Input: part model. Units: mm. Frame: model coordinates. A direction names the side the tool comes from. Coordinates: 2 decimals unless noted, no trailing zeros. Loops run counter-clockwise (first coordinate to the right, second up) from the corner with the lowest first, then second, coordinate; pieces in that order, holes last.
Item 1: Pull-direction query (Y, two-part tool) for faces 3 (the flat face through (-147, 305, 15.875)), 4 (the flat face through (165.424, 142.991, 7.826)), 5 (the flat face through (155.993, 141.57, 9.392)); classes: released by +Y, released by -Y, zero draft, split by the parting line, or undercut.
Item 2: Ray query, line 1 along X through (y, z) = (147.5, 16); line 2 along Y through (x, z) = (25, 8.75); line 3 along X through (y, z) = (29.5, 9.5). Return the intervals inside material, ascending.
Item 3: Reachability of faces 1 (the flat face through (-133.66, 416.26, 17.44)), 2 (the flat face through (-138.43, 416.8, 7.83)) from +Z, -Z, +X, -X, +Y, -Y: full face, straight path, thin tool, end or side. Return the list, or none.
Item 4: Section A-A on y = 627. Return loops of the section in (x, z) (3 decimals), and give its area (3 significant figures).
Item 5: Contact query for flat-ended pins moving along their axis: P1, Ø4, axis at x = 102.5, z = 14.5, coming from the -Y side; P2, Ø8, axis at y = 276.5, z = 16, coming from the +X side; P3, Ø10, axis at x = 84.5, z = 12, coming from the -Y side. Output: stop coordinate, or through.
```python
from build123d import *

# Parameters (mm, degrees)
BOSS_EXTRUDE1_DEPTH = 19.05
CUT_EXTRUDE1_START  = -3.175
CUT_EXTRUDE1_DEPTH  = 3.175


# Read off the part's stored shape, not the designer's step: Cut-Extrude1
with BuildPart() as part:
    # Sketch1 → Boss-Extrude1 (new body)
    with BuildSketch(Plane.XY):
        with BuildLine():
            Line((157.234081882, 128.980548454), (154.716315658, 154.51789158))
            Line((154.716315658, 154.51789158), (164.195357535, 155.452445004))
            Line((164.195357535, 155.452445004), (166.6875, 130.175))
            add(Edge.make_bspline(
                [(0, 0), (73.666580622, 1.740675992), (181.188092361, 36.200835609), (166.6875, 130.175)],
                knots=[0, 0, 0, 0, 1, 1, 1, 1], degree=3))
            add(Edge.make_bspline(
                [(0, 0), (-73.666580622, 1.740675992), (-181.188092361, 36.200835609), (-166.6875, 130.175)],
                knots=[0, 0, 0, 0, 1, 1, 1, 1], degree=3))
            Line((-166.6875, 130.175), (-109.368223301, 711.556235093))
            Line((-109.368223301, 711.556235093), (-99.889181424, 710.621681669))
            Line((-99.889181424, 710.621681669), (-157.234081882, 128.980548454))
            add(Edge.make_bspline(
                [(0, 9.52776174), (-1.117611602, 9.555193192), (-3.340472897, 9.624755056), (-7.880039481, 9.827207732), (-13.652210416, 10.198958437), (-20.725459036, 10.840441372), (-30.303235723, 11.962316267), (-42.47749757, 13.875858033), (-57.165232888, 17.02314898), (-71.689613059, 21.050850851), (-90.515854195, 27.626537064), (-112.436111514, 38.157452487), (-130.643933928, 51.803557723), (-142.189146149, 64.564536934), (-149.192253507, 75.075537554), (-153.541361304, 84.674022673), (-156.058613173, 92.923629982), (-157.442658539, 99.418206789), (-158.29640922, 106.242287005), (-158.540175044, 112.221426054), (-158.437150466, 117.190167219), (-158.20642164, 121.010360535), (-157.881730698, 124.277278241), (-157.584058118, 126.601085874), (-157.415798733, 127.781927866), (-157.316566229, 128.446705395), (-157.261207353, 128.804756083), (-157.234081882, 128.980548454)],
                knots=[0.001057036, 0.001057036, 0.001057036, 0.001057036, 0.016679825, 0.032302613, 0.063548191, 0.094793768, 0.126039346, 0.1885305, 0.251021655, 0.31351281, 0.376003965, 0.500986274, 0.625968584, 0.688459739, 0.750950893, 0.813442048, 0.844687626, 0.875933203, 0.90717878, 0.938424358, 0.954047147, 0.969669935, 0.985292724, 0.993104118, 0.997009815, 0.998962664, 1.000915513, 1.000915513, 1.000915513, 1.000915513], degree=3))
            add(Edge.make_bspline(
                [(157.234081882, 128.980548454), (157.261207353, 128.804756083), (157.316566229, 128.446705395), (157.415798733, 127.781927866), (157.584058118, 126.601085874), (157.881730698, 124.277278241), (158.20642164, 121.010360535), (158.437150466, 117.190167219), (158.540175044, 112.221426054), (158.29640922, 106.242287005), (157.442658539, 99.418206789), (156.058613173, 92.923629982), (153.541361304, 84.674022673), (149.192253507, 75.075537554), (142.189146149, 64.564536934), (130.643933928, 51.803557723), (112.436111514, 38.157452487), (90.515854195, 27.626537064), (71.689613059, 21.050850851), (57.165232888, 17.02314898), (42.47749757, 13.875858033), (30.303235723, 11.962316267), (20.725459036, 10.840441372), (13.652210416, 10.198958437), (7.880039481, 9.827207732), (3.340472897, 9.624755056), (1.117611602, 9.555193192), (0, 9.52776174)],
                knots=[0.001057036, 0.001057036, 0.001057036, 0.001057036, 0.003009885, 0.004962733, 0.00886843, 0.016679825, 0.032302613, 0.047925402, 0.063548191, 0.094793768, 0.126039346, 0.157284923, 0.1885305, 0.251021655, 0.31351281, 0.376003965, 0.500986274, 0.625968584, 0.688459739, 0.750950893, 0.813442048, 0.875933203, 0.90717878, 0.938424358, 0.969669935, 0.985292724, 1.000915513, 1.000915513, 1.000915513, 1.000915513], degree=3))
        make_face()
    extrude(amount=BOSS_EXTRUDE1_DEPTH)

    # Cut-Extrude1 outline → Cut-Extrude1 (cut)
    with BuildSketch(Plane.XY.offset(19.05).offset(CUT_EXTRUDE1_START)):
        with BuildLine():
            add(Edge.make_bspline(
                [(0, 4.801965673), (9.039076986, 5.019645615), (18.615343357, 5.740087083), (38.206551494, 8.290420977), (48.221803102, 10.120302171), (68.063126794, 14.983315661), (77.889169822, 18.016665839), (96.726604846, 25.367412999), (105.737388343, 29.685039413), (122.329339782, 39.664160586), (129.908900725, 45.324695844), (139.777007016, 54.855777785), (142.816728459, 58.206110887), (148.333510848, 65.263042796), (150.810694166, 68.969494834), (155.143109198, 76.756286204), (156.998589935, 80.836629029), (160.026646994, 89.399867478), (161.199415591, 93.883005077), (162.79196327, 103.287974059), (163.211691294, 108.210111051), (163.215151327, 115.948212654), (163.111865799, 118.586683423), (162.792061754, 122.635654517), (162.657978395, 124.000517644), (162.414585492, 126.070904339), (162.282321945, 127.11187023), (162.109292482, 128.336489493), (162.031100506, 128.86350908), (161.978072787, 129.215341168), (161.951296998, 129.389464404), (161.922977269, 129.572996421)],
                knots=[0, 0, 0, 0, 0.125, 0.125, 0.25, 0.25, 0.375, 0.375, 0.5, 0.5, 0.625, 0.625, 0.6875, 0.6875, 0.75, 0.75, 0.8125, 0.8125, 0.875, 0.875, 0.9375, 0.9375, 0.96875, 0.96875, 0.984375, 0.984375, 0.9921875, 0.99609375, 0.998046875, 0.998046875, 1, 1, 1, 1], degree=3))
            add(Edge.make_bspline(
                [(-161.922977269, 129.572996421), (-161.951296998, 129.389464404), (-161.978072787, 129.215341168), (-162.031100506, 128.86350908), (-162.109292482, 128.336489493), (-162.282321945, 127.11187023), (-162.590936716, 124.682949208), (-162.792061754, 122.635654517), (-163.111865799, 118.586683423), (-163.215151327, 115.948212654), (-163.211691294, 108.210111051), (-162.79196327, 103.287974059), (-161.199415591, 93.883005077), (-160.026646994, 89.399867478), (-156.998589935, 80.836629029), (-155.143109198, 76.756286204), (-150.810694166, 68.969494834), (-148.333510848, 65.263042796), (-142.816728459, 58.206110887), (-139.777007016, 54.855777785), (-129.908900725, 45.324695844), (-122.329339782, 39.664160586), (-105.737388343, 29.685039413), (-96.726604846, 25.367412999), (-77.889169822, 18.016665839), (-68.063126794, 14.983315661), (-48.221803102, 10.120302171), (-38.206551494, 8.290420977), (-18.615343357, 5.740087083), (-9.039076986, 5.019645615), (0, 4.801965673)],
                knots=[0, 0, 0, 0, 0.001953125, 0.001953125, 0.00390625, 0.0078125, 0.015625, 0.03125, 0.03125, 0.0625, 0.0625, 0.125, 0.125, 0.1875, 0.1875, 0.25, 0.25, 0.3125, 0.3125, 0.375, 0.375, 0.5, 0.5, 0.625, 0.625, 0.75, 0.75, 0.875, 0.875, 1, 1, 1, 1], degree=3))
            Line((-161.922977269, 129.572996421), (-104.590786195, 711.085220167))
            Line((-104.590786195, 711.085220167), (-109.368223301, 711.556235093))
            Line((-109.368223301, 711.556235093), (-166.6875, 130.175))
            add(Edge.make_bspline(
                [(-166.6875, 130.175), (-181.188092361, 36.200835609), (-73.666580622, 1.740675992), (0, 0)],
                knots=[0, 0, 0, 0, 1, 1, 1, 1], degree=3))
            add(Edge.make_bspline(
                [(0, 0), (73.666580622, 1.740675992), (181.188092361, 36.200835609), (166.6875, 130.175)],
                knots=[0, 0, 0, 0, 1, 1, 1, 1], degree=3))
            Line((166.6875, 130.175), (164.195357535, 155.452445004))
            Line((164.195357535, 155.452445004), (159.417920429, 154.981430078))
            Line((159.417920429, 154.981430078), (161.922977269, 129.572996421))
        make_face()
    extrude(amount=CUT_EXTRUDE1_DEPTH, mode=Mode.SUBTRACT)


solid = part.part
```
Results found:
1. face 3: zero draft
1. face 4: released by +Y
1. face 5: undercut
2. line 1: x = -160.16 to -155.41, 155.41 to 160.16
2. line 2: y = 1.76 to 11.35
2. line 3: x = -114.72 to -93.77, 93.77 to 114.72
3. face 1: +Z, -X, +Y
3. face 2: +Z, -Z, -X, +Y
4. outline: (-117.705, 0) - (-108.134, 0) - (-108.134, 19.05) - (-112.881, 19.05) - (-112.881, 15.875) - (-117.705, 15.875) - close
4. area: 167 mm2
5. P1: stops at y = 22.1
5. P2: stops at x = -142.3
5. P3: stops at y = 13.75
